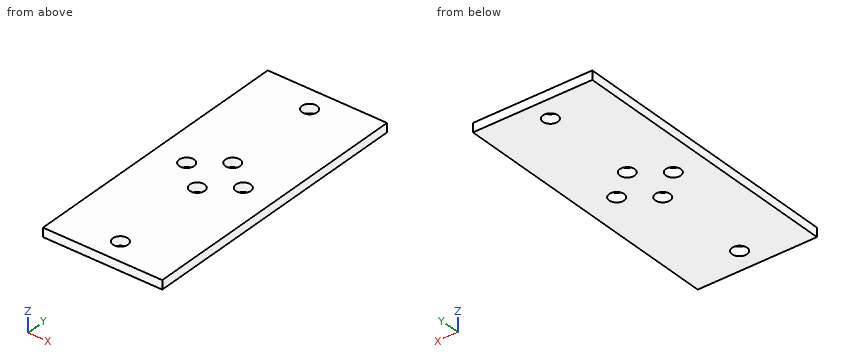
```python
from build123d import *

# Parameters (mm, degrees)
ESBO_O1_W                = 40
ESBO_O1_H                = 95
RESSALTO_EXTRUS_O1_DEPTH = 3
CUT_EXTRUDE1_REACH       = 105.121
ESBO_O2_R                = 2.5


with BuildPart() as part:
    # Esboço1 → Ressalto-extrusão1 (new body)
    with BuildSketch(Plane.XY):
        with Locations((20, 47.5)):
            Rectangle(ESBO_O1_W, ESBO_O1_H)
    extrude(amount=RESSALTO_EXTRUS_O1_DEPTH)

    # Esboço2 → Cut-Extrude1 (cut, up to next)
    with BuildSketch(Plane.XY.offset(3), mode=Mode.PRIVATE) as cut_extrude1_sk1:
        with Locations((20, 87.5)):
            Circle(ESBO_O2_R)
    cut_extrude1_tool1 = extrude(cut_extrude1_sk1.sketch, amount=-CUT_EXTRUDE1_REACH, mode=Mode.PRIVATE) & part.part
    # Esboço2 → Cut-Extrude1 (cut, up to next)
    with BuildSketch(Plane.XY.offset(3), mode=Mode.PRIVATE) as cut_extrude1_sk2:
        with Locations((20, 7.5)):
            Circle(ESBO_O2_R)
    cut_extrude1_tool2 = extrude(cut_extrude1_sk2.sketch, amount=-CUT_EXTRUDE1_REACH, mode=Mode.PRIVATE) & part.part
    # Esboço2 → Cut-Extrude1 (cut, up to next)
    with BuildSketch(Plane.XY.offset(3), mode=Mode.PRIVATE) as cut_extrude1_sk3:
        with Locations((10.5, 47.5)):
            Circle(ESBO_O2_R)
    cut_extrude1_tool3 = extrude(cut_extrude1_sk3.sketch, amount=-CUT_EXTRUDE1_REACH, mode=Mode.PRIVATE) & part.part
    # Esboço2 → Cut-Extrude1 (cut, up to next)
    with BuildSketch(Plane.XY.offset(3), mode=Mode.PRIVATE) as cut_extrude1_sk4:
        with Locations((29.5, 47.5)):
            Circle(ESBO_O2_R)
    cut_extrude1_tool4 = extrude(cut_extrude1_sk4.sketch, amount=-CUT_EXTRUDE1_REACH, mode=Mode.PRIVATE) & part.part
    # Esboço2 → Cut-Extrude1 (cut, up to next)
    with BuildSketch(Plane.XY.offset(3), mode=Mode.PRIVATE) as cut_extrude1_sk5:
        with Locations((20, 55)):
            Circle(ESBO_O2_R)
    cut_extrude1_tool5 = extrude(cut_extrude1_sk5.sketch, amount=-CUT_EXTRUDE1_REACH, mode=Mode.PRIVATE) & part.part
    # Esboço2 → Cut-Extrude1 (cut, up to next)
    with BuildSketch(Plane.XY.offset(3), mode=Mode.PRIVATE) as cut_extrude1_sk6:
        with Locations((20, 40)):
            Circle(ESBO_O2_R)
    cut_extrude1_tool6 = extrude(cut_extrude1_sk6.sketch, amount=-CUT_EXTRUDE1_REACH, mode=Mode.PRIVATE) & part.part
    add(cut_extrude1_tool1.solids().sort_by_distance((20, 87.5, 3))[0], mode=Mode.SUBTRACT)
    add(cut_extrude1_tool2.solids().sort_by_distance((20, 7.5, 3))[0], mode=Mode.SUBTRACT)
    add(cut_extrude1_tool3.solids().sort_by_distance((10.5, 47.5, 3))[0], mode=Mode.SUBTRACT)
    add(cut_extrude1_tool4.solids().sort_by_distance((29.5, 47.5, 3))[0], mode=Mode.SUBTRACT)
    add(cut_extrude1_tool5.solids().sort_by_distance((20, 55, 3))[0], mode=Mode.SUBTRACT)
    add(cut_extrude1_tool6.solids().sort_by_distance((20, 40, 3))[0], mode=Mode.SUBTRACT)


solid = part.part
```
Model file for the job. Use its own axes, mm. Give positions to 0.01 mm unless a question says otherwise; leave off trailing zeros. Loops run counter-clockwise (first coordinate to the right, second up) from the corner with the lowest first, then second, coordinate; pieces in that order, holes last. Notation, with made-up numbers: (-23.5, -34.5) -> (-12.5, -34.5) arc R17 cw to (-12.5, -18.5) -> close; hole circle Ø4 at (39.25, 22.25). An arc over 180 degrees is marked (long way). Write each question's results on one line, items separated by ' | '.
(1) Cut at B-B on y = 47.5. List the corners of the cut face in (x, z).
Geometry results:
outline: (0, 0) -> (8, 0) -> (8, 3) -> (0, 3) -> close; (13, 0) -> (27, 0) -> (27, 3) -> (13, 3) -> close; (32, 0) -> (40, 0) -> (40, 3) -> (32, 3) -> close
(2) Cut at A-A on z = 2.4. List the corners of the cut face in (x, y), and give its area (3 significant figures).
Geometry results:
outline: (0, 0) -> (40, 0) -> (40, 95) -> (0, 95) -> close; hole circle Ø5 at (10.5, 47.5); hole circle Ø5 at (20, 7.5); hole circle Ø5 at (20, 40); hole circle Ø5 at (20, 55); hole circle Ø5 at (20, 87.5); hole circle Ø5 at (29.5, 47.5) | area: 3,680 mm²
(3) Flat gauge pins, fed straight in: pin 1 Ø4 at (x, y) = (10.5, 47.5) entering from -Z; pin 2 Ø6 at (x, y) = (29.5, 47.5) entering from +Z. Where does each tip first touch, or does it go through?
Geometry results:
pin 1: passes through | pin 2: stops at z = 3
(4) Probe line 1 along Y through (x, z) = (20, 1.2); line 2 along Y through (x, z) = (29.5, 2.4); line 3 along Y through (x, z) = (31.5, 0.55). List the from-to ranges inside material, lowest first.
Geometry results:
line 1: y = 0 to 5, 10 to 37.5, 42.5 to 52.5, 57.5 to 85, 90 to 95 | line 2: y = 0 to 45, 50 to 95 | line 3: y = 0 to 46, 49 to 95
(5) Cut at C-C on x = 12. List the corners of the cut face in (y, z), and give its area (3 significant figures).
Geometry results:
outline: (0, 0) -> (45.5, 0) -> (45.5, 3) -> (0, 3) -> close; (49.5, 0) -> (95, 0) -> (95, 3) -> (49.5, 3) -> close | area: 273 mm²
(6) Cut at D-D on y = 87.5. List the corners of the cut face in (x, z).
Geometry results:
outline: (0, 0) -> (17.5, 0) -> (17.5, 3) -> (0, 3) -> close; (22.5, 0) -> (40, 0) -> (40, 3) -> (22.5, 3) -> close
